Can you work these out from the model? Positions are in its coordinate system, mm. A direction names the side the tool comes from. Give positions to 0.01 mm unless a question says otherwise; leave off trailing zeros. Order: outer loops, then holes, each group sorted by start corner. A loop starts at its lowest first (then second) coordinate and runs counter-clockwise, first axis right, second up. Notation, with made-up numbers: (11, 48) -> (67, 48) arc R22 ccw to (67, 78) -> close; hole circle Ø7 at (8.25, -14.5). An arc over 180 degrees is marked (long way). Answer as a JSON object with one key per item and string values.
```python
from build123d import *

# Parameters (mm, degrees)
BOSS_EXTRUDE1_DEPTH = 3
SKETCH1_3_W         = 3
SKETCH1_3_H         = 110
BOSS_EXTRUDE2_DEPTH = 20
SKETCH4_W           = 110
SKETCH4_H           = 3
BOSS_EXTRUDE3_DEPTH = 22
SKETCH9_W           = 153.774265812
SKETCH9_H           = 63.565026257
CUT_EXTRUDE1_DEPTH  = 15.790377159
CUT_EXTRUDE2_DEPTH  = 22
CUT_EXTRUDE3_DEPTH  = 22


with BuildPart() as part:
    # Sketch1 → Boss-Extrude1 (new body)
    with BuildSketch(Plane(origin=(0, 0, 0), x_dir=(1, 0, 0), z_dir=(0, 1, 0))):
        with BuildLine():
            Line((-25, 55), (-57, 55))
            Line((-57, 55), (-57, -55))
            Line((-57, -55), (57, -55))
            Line((57, -55), (57, 55))
            Line((57, 55), (25, 55))
            Line((25, 55), (25, 0))
            ThreePointArc((25, 0), (0, -25), (-25, 0))
            Line((-25, 0), (-25, 55))
        make_face()
    extrude(amount=BOSS_EXTRUDE1_DEPTH)

    # Sketch1_3 → Boss-Extrude2 (add)
    with BuildSketch(Plane(origin=(0, 0, 0), x_dir=(1, 0, 0), z_dir=(0, 1, 0))):
        with Locations((-58.5, 0)):
            Rectangle(SKETCH1_3_W, SKETCH1_3_H)
        with Locations((58.5, 0)):
            Rectangle(SKETCH1_3_W, SKETCH1_3_H)
    extrude(amount=BOSS_EXTRUDE2_DEPTH)

    # Sketch4 → Boss-Extrude3 (add)
    with BuildSketch(Plane(origin=(-57, 0, 0), x_dir=(0, 0, -1), z_dir=(1, 0, 0))):
        with Locations((0, 18.5)):
            Rectangle(SKETCH4_W, SKETCH4_H)
    boss_extrude3 = extrude(amount=BOSS_EXTRUDE3_DEPTH)

    # Mirror1: Boss-Extrude3 across plane
    add(boss_extrude3.mirror(Plane(origin=(0, 0, 0), x_dir=(0, 0, 1), z_dir=(1, 0, 0))))

    # Sketch9 → Cut-Extrude1 (cut, through all)
    with BuildSketch(Plane(origin=(0, 25.862068966, -14.655172414), x_dir=(1, 0, 0), z_dir=(0, 0.870022186, -0.493012572))):
        with Locations((-2.934476774, 31.782513129)):
            Rectangle(SKETCH9_W, SKETCH9_H)
    extrude(amount=CUT_EXTRUDE1_DEPTH, mode=Mode.SUBTRACT)

    # Sketch10 → Cut-Extrude2 (cut)
    with BuildSketch(Plane(origin=(0, 3, 0), x_dir=(1, 0, 0), z_dir=(0, 1, 0))):
        with BuildLine():
            Line((-36, 42.9741892), (-36, 32.9741892))
            ThreePointArc((-36, 32.9741892), (-40, 28.9741892), (-44, 32.9741892))
            Line((-44, 32.9741892), (-44, 42.9741892))
            ThreePointArc((-44, 42.9741892), (-40, 46.9741892), (-36, 42.9741892))
        make_face()
    cut_extrude2 = extrude(amount=-CUT_EXTRUDE2_DEPTH, mode=Mode.SUBTRACT)

    # Mirror2: Cut-Extrude2 across plane
    add(cut_extrude2.mirror(Plane(origin=(0, 0, 0), x_dir=(0, 0, 1), z_dir=(1, 0, 0))), mode=Mode.SUBTRACT)

    # Sketch11 → Cut-Extrude3 (cut)
    with BuildSketch(Plane(origin=(0, 3, 0), x_dir=(1, 0, 0), z_dir=(0, 1, 0))):
        with BuildLine():
            Line((4, -32), (4, -42))
            ThreePointArc((4, -42), (0, -46), (-4, -42))
            Line((-4, -42), (-4, -32))
            ThreePointArc((-4, -32), (0, -28), (4, -32))
        make_face()
    extrude(amount=-CUT_EXTRUDE3_DEPTH, mode=Mode.SUBTRACT)


solid = part.part
```
1. If we section it at C-C on x = -40: Please give me the cut outline in (y, z).
Worked answers:
{"outline": "(0, -55) -> (3, -55) -> (3, -46.97) -> (0, -46.97) -> close; (0, -28.97) -> (3, -28.97) -> (3, 55) -> (0, 55) -> close; (17, -30.29) -> (20, -25) -> (20, 55) -> (17, 55) -> close"}
2. Will this pin go through, and if not, where does the flat tip stop? pin 1 Ø8 at (x, y) = (4.5, 3.5) entering from -Z.
Worked answers:
{"pin 1": "z = 23.52"}
3. If we section it at D-D on y = 14: Please give me the cut outline in (x, z).
Worked answers:
{"outline": "(-60, -35.59) -> (-57, -35.59) -> (-57, 55) -> (-60, 55) -> close; (57, -35.59) -> (60, -35.59) -> (60, 55) -> (57, 55) -> close"}
4. If we section it at A-A on z = -11: Please give me the cut outline in (x, y), then the cut area to 3 significant figures.
Worked answers:
{"outline": "(-60, 0) -> (-25, 0) -> (-25, 3) -> (-57, 3) -> (-57, 17) -> (-35, 17) -> (-35, 20) -> (-60, 20) -> close; (25, 0) -> (60, 0) -> (60, 20) -> (35, 20) -> (35, 17) -> (57, 17) -> (57, 3) -> (25, 3) -> close", "area": "444 mm²"}
5. If we section it at B-B on x = -52: Please give me the cut outline in (y, z), then the cut area to 3 significant figures.
Worked answers:
{"outline": "(0, -55) -> (3, -55) -> (3, 55) -> (0, 55) -> close; (17, -30.29) -> (20, -25) -> (20, 55) -> (17, 55) -> close", "area": "578 mm²"}
6. Please list where these lines run through material, in increasing order: L1, parallel to Y at x = 51, z = -17; L2, parallel to X at y = 14.5, z = -25; L3, parallel to X at y = 1, z = -24.5.
Worked answers:
{"L1": "0 to 3, 17 to 20", "L2": "-60 to -57, 57 to 60", "L3": "-60 to -25, 25 to 60"}
7. If we mould it in two halves opening along Z, with no side actions, what happens to faces 4 (the face through (-48, 20, 16)), 5 (the face through (0, 2, 28)), 6 (the face through (-4.2, 2.5, 55))? For each: +Z half, -Z half, draft (parallel to the pull), parting line (faces both ways), or undercut.
Worked answers:
{"face 4": "draft", "face 5": "undercut", "face 6": "+Z half"}
8. For faces 1 (the face through (-40.088, 1.521, -46.973)), 2 (the face through (25, 1, -28)), 3 (the face through (-46, 17, 13)), which set-ups out of +Z, -Z, +X, -X, +Y, -Y let a thin tool reach every point of the face, with its end or its side?
Worked answers:
{"face 1": "+Y, -Y", "face 2": "-Z, +Y, -Y", "face 3": "+Z, -Z"}
